```python
from build123d import *

# Parameters (mm, degrees)
CHAMFER_1_SIZE = 0.5


with BuildPart() as part:
    # 草图1 → 旋转1 (revolve)
    with BuildSketch(Plane.XY, mode=Mode.PRIVATE) as revolve_1_sk:
        Polygon((-15.3, 0), (0, 0), (0, 2.5), (-1, 2.5), (-1, 2.375), (-1.7, 2.375), (-1.7, 2.5), (-13.3, 2.5), (-13.3, 3), (-15.3, 3), align=None)
    revolve(revolve_1_sk.sketch.rotate(Axis((-15.3, 0, 0), (1, 0, 0)), 90), axis=Axis((-15.3, 0, 0), (1, 0, 0)))

    # 倒角1
    chamfer_1_edges = [part.edges().sort_by_distance(p)[0] for p in [
        (0, 0, -2.5),
    ]]
    chamfer(chamfer_1_edges, length=CHAMFER_1_SIZE)


solid = part.part
```
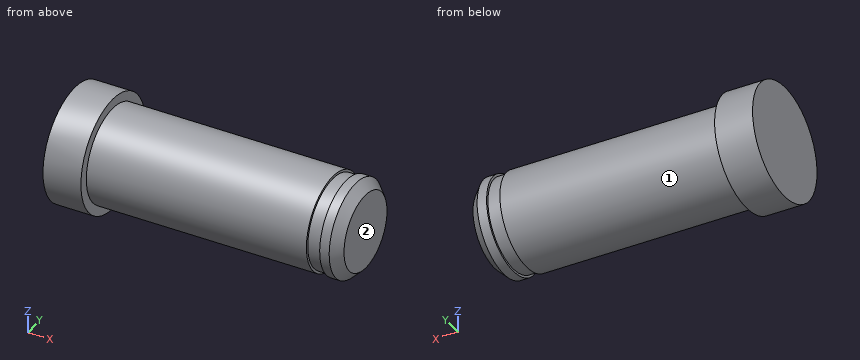
Check sheet for the modelled part. Datum: model origin and axes. Units: mm. Face numbers are marked on the shaded views. A direction names the side the tool comes from. Round coordinates to 2 decimals unless told otherwise and drop trailing zeros. Loops run counter-clockwise (first coordinate to the right, second up) from the corner with the lowest first, then second, coordinate; pieces in that order, holes last. Notation, with made-up numbers: (-33.75, -30) - (18.25, -30) arc R27 cw to (18.25, -12) - close; hole circle Ø5 at (88, 82.25). An arc over 180 degrees is marked (long way). Answer as a JSON object with one key per item and string values. Group by question number.
Q1. Scan lines: line 1 along Y through (x, z) = (-13.5, -2.25); line 2 along Y through (x, z) = (-14, -1.95); line 3 along Z through (x, y) = (-11.5, 1.9). Record each from-to range of solid material in increasing order. Write a range as [from, to].
Q2. Sectioned sample at A-A, the plane z = 0. Enter the section's corners in (x, y) (3 decimals), plus the area to 3 significant figures.
Q3. Gauge pin test, flat ends, axial feed: P1, Ø1.5, axis at x = -12, y = 1.5, coming from the +Z side; P2, Ø1.5, axis at x = -9, z = -0.5, coming from the +Y side; P3, Ø1, axis at y = -2, z = 2, coming from the +X side. Record the tip position at first contact, or that the pin passes through.
Q4. Sectioned sample at C-C, the plane x = -4.75. Enter the section's corners in (y, z), plus the area to 3 significant figures.
Q5. Set-up check for the marked faces 1 and 2: record each of +Z, -Z, +X, -X, +Y, -Y from which the full face is reachable in a straight line by a thin tool's end or side.
Solution:
{
 "1": {"line 1": "y = [-1.98, 1.98]", "line 2": "y = [-2.28, 2.28]", "line 3": "z = [-1.62, 1.62]"},
 "2": {"outline": "(-15.3, -3) - (-13.3, -3) - (-13.3, -2.5) - (-1.7, -2.5) - (-1.7, -2.375) - (-1, -2.375) - (-1, -2.5) - (-0.5, -2.5) - (0, -2) - (0, 2) - (-0.5, 2.5) - (-1, 2.5) - (-1, 2.375) - (-1.7, 2.375) - (-1.7, 2.5) - (-13.3, 2.5) - (-13.3, 3) - (-15.3, 3) - close", "area": "78.1 mm²"},
 "3": {"P1": "stops at z = 2.38", "P2": "stops at y = 2.5", "P3": "stops at x = -0.33"},
 "4": {"outline": "circle Ø5 at (0, 0)", "area": "19.6 mm²"},
 "5": {"face 1": "+X", "face 2": "+Z, -Z, +X, +Y, -Y"}
}
